from build123d import *

# Parameters (mm, degrees)
SKETCH1_W           = 17.5
SKETCH1_H           = 4
BOSS_EXTRUDE1_DEPTH = 7
CUT_EXTRUDE1_REACH  = 13.383
SKETCH3_R           = 0.75


with BuildPart() as part:
    # Sketch1 → Boss-Extrude1 (new body)
    with BuildSketch(Plane.XY):
        Rectangle(SKETCH1_W, SKETCH1_H)
    extrude(amount=-BOSS_EXTRUDE1_DEPTH)

    # Sketch3 → Cut-Extrude1 (cut, up to next)
    with BuildSketch(Plane.XY, mode=Mode.PRIVATE) as cut_extrude1_sk1:
        with Locations((-4.75, 0)):
            Circle(SKETCH3_R)
    cut_extrude1_tool1 = extrude(cut_extrude1_sk1.sketch, amount=-CUT_EXTRUDE1_REACH, mode=Mode.PRIVATE) & part.part
    # Sketch3 → Cut-Extrude1 (cut, up to next)
    with BuildSketch(Plane.XY, mode=Mode.PRIVATE) as cut_extrude1_sk2:
        with Locations((4.75, 0)):
            Circle(SKETCH3_R)
    cut_extrude1_tool2 = extrude(cut_extrude1_sk2.sketch, amount=-CUT_EXTRUDE1_REACH, mode=Mode.PRIVATE) & part.part
    add(cut_extrude1_tool1.solids().sort_by_distance((-4.75, 0, 0))[0], mode=Mode.SUBTRACT)
    add(cut_extrude1_tool2.solids().sort_by_distance((4.75, 0, 0))[0], mode=Mode.SUBTRACT)


solid = part.part
Design review of the part built by this model. Coordinates are the model's own, in mm. Round coordinates to 2 decimals unless told otherwise and drop trailing zeros. Loops run counter-clockwise (first coordinate to the right, second up) from the corner with the lowest first, then second, coordinate; pieces in that order, holes last. Notation, with made-up numbers: (31.25, 21) - (35.25, 21) arc R26 ccw to (35.25, 51) - close; hole circle Ø4 at (23, 80). An arc over 180 degrees is marked (long way). One line per question, with ' | ' between items.
1. For L1, parallel to X at y = -0.5, z = -1.25; L2, parallel to Y at x = -4.75, z = -1.75; L3, parallel to X at y = 0.25, z = -1.75, list the stretches that pass through material, from the lowest coordinate up. Write a range as [from, to].
Results are:
L1: x = [-8.75, -5.31], [-4.19, 4.19], [5.31, 8.75] | L2: y = [-2, -0.75], [0.75, 2] | L3: x = [-8.75, -5.46], [-4.04, 4.04], [5.46, 8.75]
2. Draft analysis for pull direction X (two halves, no side actions). For faces 1 (the face through (0, 0, 0)), 2 (the face through (-5.5, 0, -3.5)), 3 (the face through (-8.75, 0, -3)), state which applies: released by +X, released by -X, zero draft, split by the parting line, or undercut.
Results are:
face 1: zero draft | face 2: undercut | face 3: released by -X
3. We need section A-A, the plane y = 0. State the section outline as (x, z) points, and give its area (4 significant figures).
Results are:
outline: (-8.75, -7) - (-5.5, -7) - (-5.5, 0) - (-8.75, 0) - close; (-4, -7) - (4, -7) - (4, 0) - (-4, 0) - close; (5.5, -7) - (8.75, -7) - (8.75, 0) - (5.5, 0) - close | area: 101.5 mm²
4. We need section C-C, the plane z = -2. State the section outline as (x, y) points, and give its area (3 significant figures).
Results are:
outline: (-8.75, -2) - (8.75, -2) - (8.75, 2) - (-8.75, 2) - close; hole circle Ø1.5 at (-4.75, 0); hole circle Ø1.5 at (4.75, 0) | area: 66.5 mm²
5. We need section B-B, the plane x = 4.75. State the section outline as (y, z) points, and give its area (3 significant figures).
Results are:
outline: (-2, -7) - (-0.75, -7) - (-0.75, 0) - (-2, 0) - close; (0.75, -7) - (2, -7) - (2, 0) - (0.75, 0) - close | area: 17.5 mm²
